```python
from build123d import *

# Parameters (mm, degrees)
SKETCH_1_W          = 300
SKETCH_1_H          = 44.73
EXTRUDE_1_DEPTH     = 15
CUT_EXTRUDE_4_REACH = 305.687
EXTRUDE_START       = -15
SKETCH_6_R          = 10
EXTRUDE_2_DEPTH     = 10
SKETCH_7_R          = 1
CUT_EXTRUDE_6_DEPTH = 5
EXTRUDE_5_DEPTH     = 15
CUT_EXTRUDE_7_DEPTH = 15
SKETCH_11_R         = 12
SKETCH_11_R_2       = 10
EXTRUDE_6_DEPTH     = 3


with BuildPart() as part:
    # 草图1 → 凸台-拉伸1 (new body)
    with BuildSketch(Plane.XY):
        with Locations((150, 22.365)):
            Rectangle(SKETCH_1_W, SKETCH_1_H)
    extrude(amount=EXTRUDE_1_DEPTH)

    # 草图4 → 切除-拉伸4 (cut, up to next)
    with BuildSketch(Plane.XY.offset(15), mode=Mode.PRIVATE) as cut_extrude_4_sk1:
        with BuildLine():
            Line((300, 44.73), (153.211623388, 44.73))
            ThreePointArc((153.211623388, 44.73), (175.576623388, 22.365), (153.211623388, 0))
            Line((153.211623388, 0), (300, 0))
            Line((300, 0), (300, 44.73))
        make_face()
    cut_extrude_4_tool1 = extrude(cut_extrude_4_sk1.sketch, amount=-CUT_EXTRUDE_4_REACH, mode=Mode.PRIVATE) & part.part
    add(cut_extrude_4_tool1.solids().sort_by_distance((235.292113, 22.365, 15))[0], mode=Mode.SUBTRACT)

    # 草图6 → 凸台-拉伸2 (add)
    with BuildSketch(Plane(origin=(0, 0, 0), x_dir=(-1, 0, 0), z_dir=(0, 0, -1)).offset(EXTRUDE_START)):
        with Locations((-153.211623388, 22.365)):
            Circle(SKETCH_6_R)
    extrude(amount=-EXTRUDE_2_DEPTH)

    # 草图7 → 切除-拉伸6 (cut)
    with BuildSketch(Plane.XY.offset(25)):
        with Locations((153.211623388, 29.365)):
            Circle(SKETCH_7_R)
        with Locations((160.211623388, -284.058246776)):
            Circle(SKETCH_7_R)
        with Locations((-153.211623388, -291.058246776)):
            Circle(SKETCH_7_R)
        with Locations((-160.211623388, 22.365)):
            Circle(SKETCH_7_R)
        with Locations((160.211623388, 22.365)):
            Circle(SKETCH_7_R)
        with Locations((153.211623388, 15.365)):
            Circle(SKETCH_7_R)
        with Locations((146.211623388, 22.365)):
            Circle(SKETCH_7_R)
    extrude(amount=-CUT_EXTRUDE_6_DEPTH, mode=Mode.SUBTRACT)

    # 草图9 → 凸台-拉伸5 (add)
    with BuildSketch(Plane.XY):
        Polygon((32.615717085, -34.763598368), (82.263280801, 0), (32.615717085, 0), align=None)
    extrude(amount=EXTRUDE_5_DEPTH)

    # 草图10 → 切除-拉伸7 (cut)
    with BuildSketch(Plane(origin=(0, 0, 0), x_dir=(-1, 0, 0), z_dir=(0, 0, -1))):
        with BuildLine():
            Line((-32.615717085, 19.841648987), (-32.615717085, 0))
            Line((-32.615717085, 0), (0, 0))
            Line((0, 0), (0, 44.73))
            Line((0, 44.73), (-75.211623388, 44.73))
            ThreePointArc((-75.211623388, 44.73), (-68.486338182, 43.694879603), (-62.383586389, 40.685335471))
            Line((-62.383586389, 40.685335471), (-32.615717085, 19.841648987))
        make_face()
    extrude(amount=-CUT_EXTRUDE_7_DEPTH, mode=Mode.SUBTRACT)

    # 草图11 → 凸台-拉伸6 (add)
    with BuildSketch(Plane(origin=(0, 0, 0), x_dir=(-1, 0, 0), z_dir=(0, 0, -1)).offset(EXTRUDE_START)):
        with Locations((-153.211623388, 22.365)):
            Circle(SKETCH_11_R)
        with Locations((-153.211623388, 22.365)):
            Circle(SKETCH_11_R_2, mode=Mode.SUBTRACT)
    extrude(amount=-EXTRUDE_6_DEPTH)


solid = part.part
```
For this review, take the finished solid that the model builds, in its own axes (mm). A direction names the side the tool comes from. Coordinates: 2 decimals unless noted, no trailing zeros. Order: outer loops, then holes, each group sorted by start corner. A loop starts at its lowest first (then second) coordinate and runs counter-clockwise, first axis right, second up. Notation, with made-up numbers: (48, 76) - (96, 76) arc R15 ccw to (96, 83) - close; hole circle Ø2 at (28.25, 74). An arc over 180 degrees is marked (long way). Answer as a JSON object with one key per item and string values. Group by question number.
1. We need section D-D on y = -17.5. State the section outline as (x, z) points.
2. We need section B-B on x = 103. State the section outline as (y, z) points, then the cut area to 3 significant figures.
3. For probe 1 along Z at (x, y) = (79.5, 21.5); probe 2 along Y at (x, z) = (98, 12.5); probe 3 along X at (y, z) = (22, 18.75), list the stretches that pass through material, from the lowest coordinate up.
4. Clearance check with flat-ended pins moving along their axes: P1, Ø2, axis at y = 33.5, z = 5, coming from the -X side; P2, Ø10, axis at x = 142.5, z = 7.5, coming from the -Y side; P3, Ø0.6, axis at x = 146.5, y = 22, coming from the +Z side; P4, Ø4, axis at x = 124.5, z = 17.5, coming from the -Y side. State where each tip first meets the part, or that it passes through.
5. For faces 1 (the flat face through (117, 0, 7)), 2 (the flat face through (47.71, 30.41, 7.4)), 3 (the flat face through (155.9, 32.2, 18)), list the 3-axis set-ups (+Z, -Z, +X, -X, +Y, -Y) from which the entire face can be reached by the end or side of a thin tool; tool diameter is ignored.
6. We need section A-A on z = 2.75. State the section outline as (x, y) points (3 decimals).
7. We need section C-C on z = 22.25. State the section outline as (x, y) points (3 decimals).
Final values:
{
 "1": {"outline": "(32.62, 0) - (57.27, 0) - (57.27, 15) - (32.62, 15) - close"},
 "2": {"outline": "(0, 0) - (44.73, 0) - (44.73, 15) - (0, 15) - close", "area": "671 mm²"},
 "3": {"probe 1": "0 to 15", "probe 2": "0 to 44.73", "probe 3": "143.22 to 163.2"},
 "4": {"P1": "x = 50.69", "P2": "y = 0", "P3": "z = 20", "P4": "through"},
 "5": {"face 1": "+Z, -Z, +X, -Y", "face 2": "+Z, -Z, -X, +Y", "face 3": "+Z"},
 "6": {"outline": "(32.616, -34.764) - (82.263, 0) - (153.212, 0) arc R22.365 ccw to (153.212, 44.73) - (75.212, 44.73) arc R22.365 ccw to (62.384, 40.685) - (32.616, 19.842) - close"},
 "7": {"outline": "circle Ø20 at (153.212, 22.365); hole circle Ø2 at (146.212, 22.365); hole circle Ø2 at (153.212, 15.365); hole circle Ø2 at (153.212, 29.365); hole circle Ø2 at (160.212, 22.365)"}
}
